Here's the drawing with two shaded views (mm, measured from the low corner). I have some questions. Give positions to 0.01 mm unless a question says otherwise; leave off trailing zeros. Loops run counter-clockwise (first coordinate to the right, second up) from the corner with the lowest first, then second, coordinate; pieces in that order, holes last. Notation, with made-up numbers: (1, 8) - (22, 8) arc R18 ccw to (22, 26) - close; hole circle Ø8 at (-15.75, 39). An arc over 180 degrees is marked (long way). Use a Markdown table: item, result. Add a question column.
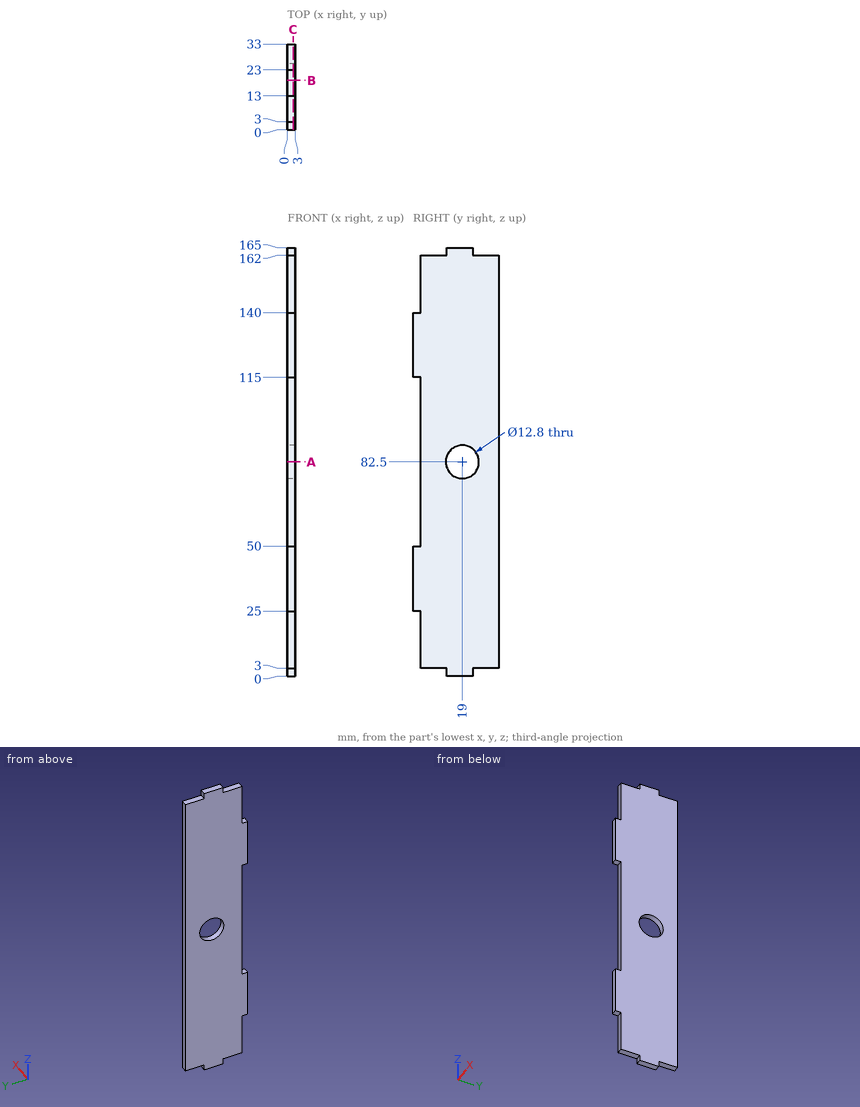
1. Suppose I cut it at C-C (x = 2.3). List the corners of the cut face in (y, z) for me, and give its area (3 significant figures).
2. Will these pins go through, and if not, where does the flat tip stop? P1, Ø1.5, axis at x = 1.5, y = 30.5, coming from the +Z side; P2, Ø1.5, axis at x = 2, y = 7.5, coming from the -Z side; P3, Ø6, axis at y = 21, z = 84.5, coming from the -X side; P4, Ø0.9, axis at x = 2, z = 1.5, coming from the +Y side.
3. Suppose I cut it at A-A (z = 82.5). List the corners of the cut face in (x, y) for me.
4. Suppose I cut it at B-B (y = 19). List the corners of the cut face in (x, z) for me.
5. Please list where these lines run through material, in increasing order: line 1 along Y through (x, z) = (0.8, 82.5); line 2 along Y through (x, z) = (2.45, 158); line 3 along Z through (x, y) = (0.5, 4). Write a range as [from, to].
Results below:
| question | item | result |
|---|---|---|
| 1 | outline | (0, 25) - (3, 25) - (3, 3) - (13, 3) - (13, 0) - (23, 0) - (23, 3) - (33, 3) - (33, 162) - (23, 162) - (23, 165) - (13, 165) - (13, 162) - (3, 162) - (3, 140) - (0, 140) - (0, 115) - (3, 115) - (3, 50) - (0, 50) - close; hole circle Ø12.8 at (19, 82.5) |
| 1 | area | 4,850 mm² |
| 2 | P1 | z = 162 |
| 2 | P2 | z = 3 |
| 2 | P3 | through |
| 2 | P4 | y = 23 |
| 3 | outline | (0, 3) - (3, 3) - (3, 12.6) - (0, 12.6) - close; (0, 25.4) - (3, 25.4) - (3, 33) - (0, 33) - close |
| 4 | outline | (0, 0) - (3, 0) - (3, 76.1) - (0, 76.1) - close; (0, 88.9) - (3, 88.9) - (3, 165) - (0, 165) - close |
| 5 | line 1 | [3, 12.6], [25.4, 33] |
| 5 | line 2 | [3, 33] |
| 5 | line 3 | [3, 162] |
